from build123d import *

# Parameters (mm, degrees)
SKETCH1_W           = 30
SKETCH1_H           = 15
SKETCH1_R           = 1
SKETCH1_R_2         = 2.38125
BOSS_EXTRUDE1_DEPTH = 9.5
SKETCH2_R           = 3
CUT_EXTRUDE1_DEPTH  = 3.5
CUT_EXTRUDE2_START  = -3
SKETCH3_R           = 3
CUT_EXTRUDE2_DEPTH  = 3


with BuildPart() as part:
    # Sketch1 → Boss-Extrude1 (new body)
    with BuildSketch(Plane.XY):
        Rectangle(SKETCH1_W, SKETCH1_H)
        Circle(SKETCH1_R, mode=Mode.SUBTRACT)
        with Locations((10, 0)):
            Circle(SKETCH1_R_2, mode=Mode.SUBTRACT)
        with Locations((-10, 0)):
            Circle(SKETCH1_R_2, mode=Mode.SUBTRACT)
    extrude(amount=BOSS_EXTRUDE1_DEPTH)

    # Sketch2 → Cut-Extrude1 (cut)
    with BuildSketch(Plane.XY.offset(9.5)):
        Circle(SKETCH2_R)
    extrude(amount=-CUT_EXTRUDE1_DEPTH, mode=Mode.SUBTRACT)

    # Sketch3 → Cut-Extrude2 (cut)
    with BuildSketch(Plane(origin=(0, 0, 0), x_dir=(-1, 0, 0), z_dir=(0, 0, -1)).offset(CUT_EXTRUDE2_START)):
        with Locations(Location((0, 0, 0), (0, 0, 180))):
            Circle(SKETCH3_R)
    extrude(amount=CUT_EXTRUDE2_DEPTH, mode=Mode.SUBTRACT)


solid = part.part
Input: part model. Units: mm. Frame: model coordinates. A direction names the side the tool comes from. Round coordinates to 2 decimals unless told otherwise and drop trailing zeros. Write each loop counter-clockwise with the first axis right and the second up, starting at its lowest first coordinate (ties: lowest second). Pieces come first, ordered by that corner, then holes.
1) Reachability of faces 5 (the flat face through (-1, 1, 6)), 6 (the flat face through (-0.2, 3.4, 0)), 7 (the flat face through (-1, -1, 3)) from +Z, -Z, +X, -X, +Y, -Y: full face, straight path, thin tool, end or side. Return the list, or none.
2) Cut plane C-C (z = 9). Return the cut outline in (x, y), then the cut area to 3 significant figures.
3) Draft query along Y for faces 1 (the cylindrical face through (7.62, 0.1, 4.68)), 2 (the cylindrical face through (2.86, -0.9, 1.52)), 3 (the flat face through (-15, 0, 5)), 4 (the flat face through (0, 7.5, 5)). Return one class per face: pulls with the +Y half, pulls with the -Y half, needs draft (parallel to the pull), parting line crosses it, or undercut.
4) Ray query, L1, parallel to X at y = 1.75, z = 1.5; L2, parallel to Y at x = 10, z = 5.75; L3, parallel to Y at x = 0, z = 3.6. Return the intervals inside material, ascending.
5) Cut plane B-B (y = 0). Return the cut outline in (x, z).
6) Contact query for flat-ended pins moving along their axis: P1, Ø3.5, axis at x = 0, y = 0, coming from the +Z side; P2, Ø1.8, axis at x = 1, y = 0, coming from the -Z side. Output: stop coordinate, or through.
7) Cut plane A-A (x = -10). Return the cut outline in (y, z), then the cut area to 3 significant figures.
8) Cut plane D-D (x = 0). Return the cut outline in (y, z).
Geometry says:
1. face 5: +Z
1. face 6: -Z, +X, -X, +Y, -Y
1. face 7: -Z
2. outline: (-15, -7.5) - (15, -7.5) - (15, 7.5) - (-15, 7.5) - close; hole circle Ø4.76 at (-10, 0); hole circle Ø6 at (0, 0); hole circle Ø4.76 at (10, 0)
2. area: 386 mm2
3. face 1: undercut
3. face 2: undercut
3. face 3: needs draft
3. face 4: pulls with the +Y half
4. L1: x = -15 to -11.61, -8.39 to -2.44, 2.44 to 8.39, 11.61 to 15
4. L2: y = -7.5 to -2.38, 2.38 to 7.5
4. L3: y = -7.5 to -1, 1 to 7.5
5. outline: (-15, 0) - (-12.38, 0) - (-12.38, 9.5) - (-15, 9.5) - close; (-7.62, 0) - (-3, 0) - (-3, 3) - (-1, 3) - (-1, 6) - (-3, 6) - (-3, 9.5) - (-7.62, 9.5) - close; (1, 3) - (3, 3) - (3, 0) - (7.62, 0) - (7.62, 9.5) - (3, 9.5) - (3, 6) - (1, 6) - close; (12.38, 0) - (15, 0) - (15, 9.5) - (12.38, 9.5) - close
6. P1: stops at z = 6
6. P2: stops at z = 3
7. outline: (-7.5, 0) - (-2.38, 0) - (-2.38, 9.5) - (-7.5, 9.5) - close; (2.38, 0) - (7.5, 0) - (7.5, 9.5) - (2.38, 9.5) - close
7. area: 97.3 mm2
8. outline: (-7.5, 0) - (-3, 0) - (-3, 3) - (-1, 3) - (-1, 6) - (-3, 6) - (-3, 9.5) - (-7.5, 9.5) - close; (1, 3) - (3, 3) - (3, 0) - (7.5, 0) - (7.5, 9.5) - (3, 9.5) - (3, 6) - (1, 6) - close
